Could you check a few things on this model? Use its own coordinates, in mm. A direction names the side the tool comes from. Round coordinates to 2 decimals unless told otherwise and drop trailing zeros. One line per item, written item: value.
Autodesk Inventor part; units mm, degrees
ref_plane "YZ Plane" through (0, 0, 0) normal (1, 0, 0) x (0, 1, 0)
ref_plane "XZ Plane" through (0, 0, 0) normal (0, 1, 0) x (-1, 0, 0)
ref_plane "XY Plane" through (0, 0, 0) normal (0, 0, 1) x (1, 0, 0)
sketch "Sketch1" plane through (0, 0, 0) normal (0, 0, 1) x (1, 0, 0)
  line L0 (0, 0) -> (-170, 0)
  line L1 (-170, 0) -> (-170, -50)
  line L2 (-170, -50) -> (0, -50)
  line L3 (0, -50) -> (0, 0)
  line L4 (0, 0) -> (-43.459, 0)
  line L5 (-43.459, 0) -> (-43.459, -8)
  line L6 (-43.459, -8) -> (0, -8)
  line L7 (0, -8) -> (0, 0)
  line L8 (0, 0) -> (-170, 0)
  line L9 (-170, 0) -> (-170, 27)
  line L10 (-170, 27) -> (0, 27)
  line L11 (0, 27) -> (0, 0)
  circle A0 centre (-50, -38) radius 4
  line L12 (-51, -30.5) -> (-49, -30.5)
  line L13 (-49, -30.5) -> (-49, -45.5)
  line L14 (-49, -45.5) -> (-51, -45.5)
  line L15 (-51, -45.5) -> (-51, -30.5)
  line L16 (-50, -38) -> (-50, -42) construction
  line L17 (-51, -38) -> (-50, -38) construction
  point P0 (-51, -34.127)
  point P1 (-51, -41.873)
  point P2 (-49, -34.127)
  point P3 (-49, -41.873)
  dimension "d10" = 8
  dimension "d0" = 43.459
  dimension "d1" = 8
  dimension "d2" = 27
  dimension "d3" = 42
  dimension "d4" = 170
  dimension "d8" = 30
  dimension "d9" = 50
  dimension "d11" = 15
  dimension "d12" = 2
sketch "Sketch2" plane through (0, 0, 0) normal (0, 0, 1) x (1, 0, 0)
  line L0 (0, 27) -> (-160, 27)
  line L1 (-160, 27) -> (-160, -50)
  line L2 (-160, -50) -> (0, -50)
  line L3 (0, -50) -> (0, 27)
  point P0 (0, 0)
  dimension "d5" = 160
extrude "Extrusion1" add sketch "Sketch2" along normal blind 5
extrude "Extrusion2" cut sketch "Sketch1" along normal through all contours A0 L13 | L13 A0 L15 | A0 L15 L12 L13 | L13 L14 L15 A0 | L15 A0
properties part number "Inkpath_Plate"
(1) On a 3-axis mill with a long thin cutter (end or side, diameter ignored), from which of +Z, -Z, +X, -X, +Y, -Y can I reach the whole of each face in a straight line? I mean faces 1 (the face through (-79, 27, 2)), 2 (the face through (-51, -44, 2)). Say none if no direction works.
Results below:
face 1: +Z, -Z, +X, -X, +Y
face 2: +Z, -Z
(2) We'd pull the mould along X, two halves only. Please class faces 3 (the face through (-160, -11, 2)), 4 (the face through (0, -12, 2)), 5 (the face through (-81, -11, 0)), 6 (the face through (-54, -38, 2)): +X half, -X half, draft (parallel to the pull), parting line (faces both ways), or undercut.
Results below:
face 3: -X half
face 4: +X half
face 5: draft
face 6: undercut
(3) For pin 1 Ø1.5 at (y, z) = (-41, 4) entering from +X, with a flat end and sliding along its axis, tell me the tip position at first contact or that it passes through.
Results below:
pin 1: stops at x = 0
(4) Please list where these lines run through material, in increasing order: L1, parallel to X at y = -34, z = 3.35; L2, parallel to Y at x = -50.5, z = 4.5; L3, parallel to X at y = -35, z = 3.2.
Results below:
L1: x = -160 to -51, -49 to 0
L2: y = -50 to -45.5, -30.5 to 27
L3: x = -160 to -52.65, -47.35 to 0
